Design review of the part built by this model. Coordinates are the model's own, in mm. A direction names the side the tool comes from. Give positions to 0.01 mm unless a question says otherwise; leave off trailing zeros. Write each loop counter-clockwise with the first axis right and the second up, starting at its lowest first coordinate (ties: lowest second). Pieces come first, ordered by that corner, then holes. Notation, with made-up numbers: (-13, 42) -> (36, 42) arc R21 ccw to (36, 55) -> close; hole circle Ø7 at (-9.75, 3). An arc over 180 degrees is marked (long way). Answer as a JSON object with one key per item and string values.
```python
from build123d import *

# Parameters (mm, degrees)
F1_DEPTH = 32
F4_D     = 8
F5_D     = 8


with BuildPart() as f1:
    # F0 (on Front) → F1 (new body)
    with BuildSketch(Plane.XZ):
        with BuildLine():
            Line((0, 37), (0, 0))
            Line((0, 0), (37, 0))
            ThreePointArc((37, 0), (34.735887, 4.452031), (30.44, 7))
            Line((30.44, 7), (10.44, 7))
            Line((10.44, 7), (7, 10.44))
            Line((7, 10.44), (7, 30.44))
            ThreePointArc((7, 30.44), (4.330611, 34.606323), (0, 37))
        make_face()
    extrude(amount=F1_DEPTH)

    # F4 (through all)
    with Locations(Plane.YZ.offset(7)):
        with Locations((-16.124548, 18.460734)):
            Hole(F4_D / 2)

    # F5 (through all)
    with Locations(Plane.XY.offset(7)):
        with Locations((17.951785, -16.037369)):
            Hole(F5_D / 2)


solid = f1.part
```
(1) We need section D-D, the plane y = -19. State the section outline as (x, z) points.
Here are the results:
{"outline": "(0, 0) -> (15.26, 0) -> (15.26, 7) -> (10.44, 7) -> (7, 10.44) -> (7, 15.68) -> (0, 15.68) -> close; (0, 21.24) -> (7, 21.24) -> (7, 30.44) arc R10.08 ccw to (0, 37) -> close; (20.64, 0) -> (37, 0) arc R8.96 ccw to (30.44, 7) -> (20.64, 7) -> close"}
(2) We need section A-A, the plane z = 15. State the section outline as (x, y) points.
Here are the results:
{"outline": "(0, -32) -> (7, -32) -> (7, -18.13) -> (0, -18.13) -> close; (0, -14.12) -> (7, -14.12) -> (7, 0) -> (0, 0) -> close"}
(3) We need section B-B, the plane y = -6. State the section outline as (x, z) points, then the cut area to 3 significant figures.
Here are the results:
{"outline": "(0, 0) -> (37, 0) arc R8.96 ccw to (30.44, 7) -> (10.44, 7) -> (7, 10.44) -> (7, 30.44) arc R10.08 ccw to (0, 37) -> close", "area": "446 mm²"}
(4) We need section C-C, the plane x = 17.5. State the section outline as (y, z) points.
Here are the results:
{"outline": "(-32, 0) -> (-20.01, 0) -> (-20.01, 7) -> (-32, 7) -> close; (-12.06, 0) -> (0, 0) -> (0, 7) -> (-12.06, 7) -> close"}
(5) The part is to be moulded in two halves that separate along Y. For faces 3 (the cylindrical face through (3.451, -13.176, 21.164)), 4 (the flat face through (22.4, -15.8, 0)), 5 (the flat face through (10, -32, 6)), say which applies: +Y half, -Y half, draft (parallel to the pull), parting line (faces both ways), or undercut.
Here are the results:
{"face 3": "undercut", "face 4": "draft", "face 5": "-Y half"}
(6) Clearance check with flat-ended pins moving along their axes: pin 1 (10 mm diameter, centred on x = 25, y = -9, fed in from +Z); pin 2 (4 mm diameter, centred on y = -15.5, z = 21, fed in from -X); pin 3 (10 mm diameter, centred on y = -12, z = 23, fed in from +X). State where each tip first meets the part, or that it passes through.
Here are the results:
{"pin 1": "stops at z = 7", "pin 2": "stops at x = 0", "pin 3": "stops at x = 7"}
(7) For faces 1 (the flat face through (7, -16, 23)), 2 (the flat face through (10, 0, 6)), list the 3-axis set-ups (+Z, -Z, +X, -X, +Y, -Y) from which the entire face can be reached by the end or side of a thin tool; tool diameter is ignored.
Here are the results:
{"face 1": "+Z, +X, +Y, -Y", "face 2": "+Z, -Z, +X, -X, +Y"}
(8) For line 1 along Z through (x, y) = (16, -29.5); line 2 along Z through (x, y) = (3, -19), list the stretches that pass through material, from the lowest coordinate up.
Here are the results:
{"line 1": "z = 0 to 7", "line 2": "z = 0 to 15.68, 21.24 to 35.66"}
